Autodesk Fusion 360 part; units mm, degrees
sketch "Sketch1" plane through (0, 0, 0) normal (0, 0, 1) x (1, 0, 0)
  line L0 (0, 0) -> (-42.5, 0)
  line L1 (-42.5, 0) -> (-42.5, 18) construction
  line L2 (-42.5, 18) -> (0, 18)
  line L3 (0, 18) -> (0, 0)
  arc A0 (-33.5, 18) -> (-33.5, 0) centre (-33.5, 9) ccw
  line L4 (-33.5, 18) -> (-29.5, 18)
  line L5 (-33.5, 0) -> (-29.5, 0)
  line L6 (-33.5, 0.5) -> (-29.5, 0.5)
  arc A1 (-33.5, 17.5) -> (-33.5, 0.5) centre (-33.5, 9) ccw
  line L7 (-33.5, 17.5) -> (-29.5, 17.5)
  line L8 (-29.5, 18) -> (-29.5, 17.5)
  line L9 (-29.5, 0.5) -> (-29.5, 0)
  dimension "d6" = 42.5
  dimension "d7" = 18
  dimension "d8" = 4
  dimension "d9" = 4
extrude "Extrude1" add sketch "Sketch1" against normal blind 0.8
extrude "Extrude2" add sketch "Sketch1" along normal blind 30 contours L0 L2 A0 L4 L5 L6 A1 L7 L8 L9
sketch "Sketch2" plane through (0, 0, 0) normal (0, -1, 0) x (1, 0, 0)
  line L0 (-33.5, 30) -> (-33.5, -0.8)
  line L1 (-33.5, -0.8) -> (0, -0.8)
  line L2 (0, -0.8) -> (0, 0)
  line L3 (0, 0) -> (-29.5, 0)
  line L4 (-29.5, 0) -> (-29.5, 30)
  line L5 (-29.5, 30) -> (-33.5, 30)
  line L6 (-33.5, 0) -> (-29.5, 0)
  line L7 (-29.5, 5.7) -> (-30.2, 5)
  line L8 (-30.2, 5) -> (-29.5, 5)
  line L9 (-29.5, 5.7) -> (-29.5, 5)
  dimension "d31" = 0.7
  dimension "d32" = 45
  dimension "d33" = 5
extrude "Extrude3" cut sketch "Sketch2" against normal through all contours L4 L7 L8 L9
pattern_linear "R-Pattern1" count 5 spacing 5 along (0, 0, 1) of "Extrude3"
mirror "Mirror1" about plane through (0, 0, 0) normal (1, 0, 0) of bodies 1 merged
sketch "Sketch3" plane through (0, 0, 0) normal (0, 0, 1) x (-1, 0, 0)
  arc A0 (-33.5, -0.5) -> (-33.5, -17.5) centre (-33.5, -9) ccw
  arc A1 (33.5, -17.5) -> (33.5, -0.5) centre (33.5, -9) ccw
  circle A2 centre (0, 0) radius 2
  line L0 (29.5, -0.5) -> (29.5, 0)
  line L1 (29.5, 0) -> (-29.5, 0)
  line L2 (-29.5, 0) -> (-29.5, -0.5)
  line L3 (-29.5, -0.5) -> (-33.5, -0.5)
  line L4 (-33.5, -17.5) -> (-29.5, -17.5)
  line L5 (-29.5, -17.5) -> (-29.5, -18)
  line L6 (-29.5, -18) -> (29.5, -18)
  line L7 (29.5, -18) -> (29.5, -17.5)
  line L8 (29.5, -17.5) -> (33.5, -17.5)
  line L9 (33.5, -0.5) -> (29.5, -0.5)
  dimension "d27" = 4
extrude "Extrude4" cut sketch "Sketch3" against normal through all contours A2 L1 picked at (1.1554, -0.8465)
fillet "Fillet1" radius 4 2 edges at (-2, 0, -0.4) (2, 0, -0.4)
equation "baseThickness = 0.8 mm"
equation "baseLength = 85 mm"
equation "baseWidth = 18 mm"
equation "segmentHeight = 5 mm"
equation "extrusionWidth = 0.5 mm"
equation "d14 = numSegments * segmentHeight"
equation "layerHeight = 0.2 mm"
equation "d21 = numSegments - 1"
equation "d23 = segmentHeight"
equation "d31 = segmentNotchHeight"
equation "d33 = segmentHeight"
equation "segmentNotchHeight = 0.7 mm"
The listing builds one solid part. Answer for the finished solid, in the listing's coordinates (mm). A direction names the side the tool comes from. Coordinates: 2 decimals unless noted, no trailing zeros. Loops run counter-clockwise (first coordinate to the right, second up) from the corner with the lowest first, then second, coordinate; pieces in that order, holes last. Notation, with made-up numbers: M 21.25,35.5 L 63.25,35.5 A20 cw 63.25,58.5 Z; hole C 18,43 d4. An arc over 180 degrees is marked long. Answer as CSV lines item,"result". Start each with the question number.
(1) The part is cut by section B-B (y = 9). Give the vertices of the cut face in (x, z), and give its area (3 significant figures).
(2) For faces 1 (the cylindrical face through (42, 9, 15)), 2 (the flat face through (-30, 0, 12)), determine the directions among +Z, -Z, +X, -X, +Y, -Y from which every point of the face is accessible in a straight line to the end or side of a thin tool.
(3) Find the intervals of material crossed by L1, parallel to Z at x = 20.5, y = 17; L2, parallel to X at y = 13, z = 9.5; L3, parallel to Y at x = 36, z = 10.5, in increasing order. Write a range as [from, to].
(4) The part is cut by section A-A (z = 2). Give the vertices of the cut face in (x, y), and give its area (3 significant figures).
(5) The mould has two halves that part along X. Classify faces 3 (the cylindrical face through (42.498, 9.198, 14.384)), 4 (the flat face through (-32, 17.5, 15)), 5 (the flat face through (-0.2, 18, -0.3)), 6 (the flat face through (31, 17.5, 15)): pulls with the +X half, pulls with the -X half, needs draft (parallel to the pull), parting line crosses it, or undercut.
(6) Given pin 1 (1 mm diameter, centred on y = 6.5, z = 5.5, fed in from +X); pin 2 (2 mm diameter, centred on x = -17, y = 11, fed in from +Z); pin 3 (4 mm diameter, centred on y = 3.5, z = 17.5, fed in from -X), each flat-ended and moving along its own axis, determine where each tip first touches the part or whether it passes through.
(7) The part is cut by section C-C (x = 0). Give the vertices of the cut face in (y, z), and give its area (3 significant figures).
(8) The part is cut by section D-D (x = 18). Give the vertices of the cut face in (y, z).
Determined:
1,outline,"M -42.5,-0.8 L 42.5,-0.8 L 42.5,30 L 42,30 L 42,0 L -42,0 L -42,30 L -42.5,30 Z"
1,area,"98.0 mm2"
2,face 1,"+Z"
2,face 2,"+Z, -Z, +X, -X, -Y"
3,L1,"[-0.8, 0]"
3,L2,"[-41.56, -41], [41, 41.56]"
3,L3,"[0.35, 0.88], [17.12, 17.65]"
4,outline,"M -33.5,0 L -29.5,0 L -29.5,0.5 L -33.5,0.5 A8.5 cw -33.5,17.5 L -29.5,17.5 L -29.5,18 L -33.5,18 A9 ccw Z; M 29.5,0 L 33.5,0 A9 ccw 33.5,18 L 29.5,18 L 29.5,17.5 L 33.5,17.5 A8.5 cw 33.5,0.5 L 29.5,0.5 Z"
4,area,"35.5 mm2"
5,face 3,"pulls with the +X half"
5,face 4,"undercut"
5,face 5,"needs draft"
5,face 6,"undercut"
6,pin 1,"x = 42.27"
6,pin 2,"z = 0"
6,pin 3,"x = -41.79"
7,outline,"M 2,-0.8 L 18,-0.8 L 18,0 L 2,0 Z"
7,area,"12.8 mm2"
8,outline,"M 0,-0.8 L 18,-0.8 L 18,0 L 0,0 Z"
